from build123d import *

# Parameters (mm, degrees)
SKETCH_1_W      = 80
SKETCH_1_H      = 31
SKETCH_1_W_2    = 61
SKETCH_1_H_2    = 12
EXTRUDE_1_DEPTH = 3
SKETCH_2_W      = 10
SKETCH_2_H      = 3
EXTRUDE_2_DEPTH = 3


with BuildPart() as part:
    # 草图1 → 凸台-拉伸1 (new body)
    with BuildSketch(Plane.XY):
        with Locations((40, 15.5)):
            Rectangle(SKETCH_1_W, SKETCH_1_H)
        with Locations((31.5, 15.5)):
            Rectangle(SKETCH_1_W_2, SKETCH_1_H_2, mode=Mode.SUBTRACT)
    extrude(amount=EXTRUDE_1_DEPTH)

    # 草图2 → 凸台-拉伸2 (add)
    with BuildSketch(Plane.XY.offset(3)):
        with Locations((16.5, 32.5)):
            Rectangle(SKETCH_2_W, SKETCH_2_H)
        with Locations((64, 32.5)):
            Rectangle(SKETCH_2_W, SKETCH_2_H)
        with Locations((64, -1.5)):
            Rectangle(SKETCH_2_W, SKETCH_2_H)
        with Locations((16.5, -1.5)):
            Rectangle(SKETCH_2_W, SKETCH_2_H)
    extrude(amount=-EXTRUDE_2_DEPTH)


solid = part.part
For this review, take the finished solid that the model builds, in its own axes (mm). A direction names the side the tool comes from. Give positions to 0.01 mm unless a question says otherwise; leave off trailing zeros. Loops run counter-clockwise (first coordinate to the right, second up) from the corner with the lowest first, then second, coordinate; pieces in that order, holes last. Notation, with made-up numbers: (-15.75, 27.5) -> (7.25, 27.5) arc R18 cw to (7.25, 53.5) -> close; hole circle Ø9 at (34, 19). An arc over 180 degrees is marked (long way). One line per question, with ' | ' between items.
1) The part is to be moulded in two halves that separate along X. For faces 1 (the flat face through (11.5, -2, 2)), 2 (the flat face through (31, 9.5, 1)), 3 (the flat face through (6, 31, 1)), say which applies: +X half, -X half, draft (parallel to the pull), parting line (faces both ways), or undercut.
Resolved:
face 1: -X half | face 2: undercut | face 3: draft
2) We need section C-C (z = 1.05). Write out the cut boundary in (x, y).
Resolved:
outline: (0, 0) -> (11.5, 0) -> (11.5, -3) -> (21.5, -3) -> (21.5, 0) -> (59, 0) -> (59, -3) -> (69, -3) -> (69, 0) -> (80, 0) -> (80, 31) -> (69, 31) -> (69, 34) -> (59, 34) -> (59, 31) -> (21.5, 31) -> (21.5, 34) -> (11.5, 34) -> (11.5, 31) -> (0, 31) -> close; hole (1, 9.5) -> (62, 9.5) -> (62, 21.5) -> (1, 21.5) -> close
3) We need section B-B (x = 43). Write out the cut boundary in (y, z), plus the area to 3 significant figures.
Resolved:
outline: (0, 0) -> (9.5, 0) -> (9.5, 3) -> (0, 3) -> close; (21.5, 0) -> (31, 0) -> (31, 3) -> (21.5, 3) -> close | area: 57.0 mm2
4) For faces 4 (the flat face through (74, 0, 1)), 5 (the flat face through (74, 31, 1)), 6 (the flat face through (1, 15, 1)), 7 (the flat face through (59, -2, 2)), list the 3-axis set-ups (+Z, -Z, +X, -X, +Y, -Y) from which the entire face can be reached by the end or side of a thin tool; tool diameter is ignored.
Resolved:
face 4: +Z, -Z, +X, -Y | face 5: +Z, -Z, +X, +Y | face 6: +Z, -Z | face 7: +Z, -Z, -Y
5) Insertion check: pin 1 Ø1.5 at (y, z) = (-1, 2) entering from -X; pin 2 Ø1.5 at (y, z) = (33, 2) entering from +X; pin 3 Ø1.5 at (x, z) = (37.5, 1.5) entering from +Y. Each pin has a flat end and moves straight along its axis. Give the tip position at first contact, or say it passes through.
Resolved:
pin 1: stops at x = 11.5 | pin 2: stops at x = 69 | pin 3: stops at y = 31
6) We need section A-A (y = 13). Write out the cut boundary in (x, z), plus the area to 3 significant figures.
Resolved:
outline: (0, 0) -> (1, 0) -> (1, 3) -> (0, 3) -> close; (62, 0) -> (80, 0) -> (80, 3) -> (62, 3) -> close | area: 57.0 mm2
7) To check wall thickness, follow probe 1 along X at (y, z) = (15, 0.4); probe 2 along Y at (x, z) = (4.5, 1.3); probe 3 along X at (y, z) = (-0.5, 0.85). State the ranges of each line that lie inside material, in increasing order.
Resolved:
probe 1: x = 0 to 1, 62 to 80 | probe 2: y = 0 to 9.5, 21.5 to 31 | probe 3: x = 11.5 to 21.5, 59 to 69
